Here's how the part is built. I have some questions about the finished solid (model axes, mm). A direction names the side the tool comes from. Round coordinates to 2 decimals unless told otherwise and drop trailing zeros. Write each loop counter-clockwise with the first axis right and the second up, starting at its lowest first coordinate (ties: lowest second). Pieces come first, ordered by that corner, then holes. Notation, with made-up numbers: (51, 77.5) -> (70, 77.5) arc R31 cw to (70, 102.5) -> close; hole circle Ø11 at (78, 60). An arc over 180 degrees is marked (long way). Put each result on its own line as item: value. Start each with the question number.
1) Which directions (+Z, -Z, +X, -X, +Y, -Y) give clear straight access to the entire face, cutting with the end or side of a thin tool? Please do faces 4 (the flat face through (225, -9, 114.3)), 5 (the flat face through (135, -10, 25.4)), 6 (the flat face through (164, -10, 44.45)).
2) If I drill on line 1 along Z through (x, y) = (111.5, -16.75); line 2 along X through (y, z) = (-14.5, 50.8) (3 decimals); line 3 along X through (y, z) = (-16, 80), over which ranges is the centre line in solid material (lowest first)? Write a range as [from, to].
3) We'd pull the mould along X, two halves only. Please class faces 1 (the flat face through (0, -9, 56)), 2 (the flat face through (95.25, -10, 85)), 3 (the flat face through (135, 0, 20)): released by +X, released by -X, zero draft, split by the parting line, or undercut.
4) I want a section at D-D, the plane z = 50.8. List the corners of the cut face in (x, y) for me (3 decimals), then the cut area to 3 significant figures.
5) I want a section at A-A, the plane z = 80. List the corners of the cut face in (x, y) for me.
6) Will these pins go through, and if not, where does the flat tip stop? P1, Ø3, axis at y = -13, z = 39, coming from the -X side; P2, Ø8.5, axis at x = 110, y = -5.5, coming from the +Z side.
7) I want a section at B-B, the plane x = 32.5. List the corners of the cut face in (y, z) for me.
8) I want a section at C-C, the plane y = -5.5. List the corners of the cut face in (x, z) for me (3 decimals).
from build123d import *

# Parameters (mm, degrees)
F0_W     = 273.05
F0_H     = 114.3
F1_DEPTH = 19.05
F2_R     = 25.4
F3_DEPTH = 25.4
F5_DEPTH = 25.4
F7_DEPTH = 25.4


with BuildPart() as f1:
    # F0 (on Front) → F1 (new body)
    with BuildSketch(Plane.XZ):
        with Locations((136.525, 57.15)):
            Rectangle(F0_W, F0_H)
    extrude(amount=F1_DEPTH)

    # F2 (on face) → F3 (cut)
    with BuildSketch(Plane.XZ.offset(19.05)):
        with Locations((225.425, 50.8)):
            Circle(F2_R)
        with Locations((47.625, 50.8)):
            Circle(F2_R)
    extrude(amount=-F3_DEPTH, mode=Mode.SUBTRACT)

    # F4 (on face) → F5 (cut)
    with BuildSketch(Plane.XZ.offset(19.05)):
        with BuildLine():
            Line((177.8, 114.3), (95.25, 114.3))
            Line((95.25, 114.3), (95.25, 55.88))
            ThreePointArc((95.25, 55.88), (98.597769, 47.797769), (106.68, 44.45))
            Line((106.68, 44.45), (166.37, 44.45))
            ThreePointArc((166.37, 44.45), (174.452231, 47.797769), (177.8, 55.88))
            Line((177.8, 55.88), (177.8, 114.3))
        make_face()
    extrude(amount=-F5_DEPTH, mode=Mode.SUBTRACT)

    # F6 (on face) → F7 (cut)
    with BuildSketch(Plane.XZ.offset(19.05)):
        Polygon((117.475, 34.951167), (67.473791, 34.951167), (47.625, 25.4), (225.425, 25.4), (205.576209, 34.951167), (166.37, 34.951167), (161.29, 34.951167), (161.29, 44.45), (117.475, 44.45), align=None)
    extrude(amount=-F7_DEPTH, mode=Mode.SUBTRACT)


solid = f1.part
Findings:
1. face 4: +Z, +X, -X, +Y, -Y
1. face 5: +Y, -Y
1. face 6: +Z, +Y, -Y
2. line 1: z = [0, 25.4], [34.95, 44.45]
2. line 2: x = [0, 22.225], [73.025, 96.441], [176.609, 200.025], [250.825, 273.05]
2. line 3: x = [0, 95.25], [177.8, 273.05]
3. face 1: released by -X
3. face 2: undercut
3. face 3: zero draft
4. outline: (0, -19.05) -> (22.225, -19.05) -> (22.225, 0) -> (0, 0) -> close; (73.025, -19.05) -> (96.441, -19.05) -> (96.441, 0) -> (73.025, 0) -> close; (176.609, -19.05) -> (200.025, -19.05) -> (200.025, 0) -> (176.609, 0) -> close; (250.825, -19.05) -> (273.05, -19.05) -> (273.05, 0) -> (250.825, 0) -> close
4. area: 1,740 mm2
5. outline: (0, -19.05) -> (95.25, -19.05) -> (95.25, 0) -> (0, 0) -> close; (177.8, -19.05) -> (273.05, -19.05) -> (273.05, 0) -> (177.8, 0) -> close
6. P1: stops at x = 0
6. P2: stops at z = 44.49
7. outline: (-19.05, 0) -> (0, 0) -> (0, 30.39) -> (-19.05, 30.39) -> close; (-19.05, 71.21) -> (0, 71.21) -> (0, 114.3) -> (-19.05, 114.3) -> close
8. outline: (0, 0) -> (273.05, 0) -> (273.05, 114.3) -> (177.8, 114.3) -> (177.8, 55.88) arc R11.43 cw to (166.37, 44.45) -> (161.29, 44.45) -> (161.29, 34.951) -> (205.576, 34.951) arc R25.4 cw (long way) to (225.425, 25.4) -> (47.625, 25.4) arc R25.4 cw (long way) to (67.474, 34.951) -> (117.475, 34.951) -> (117.475, 44.45) -> (106.68, 44.45) arc R11.43 cw to (95.25, 55.88) -> (95.25, 114.3) -> (0, 114.3) -> close
